from build123d import *

# Parameters (mm, degrees)
SKETCH1_W                      = 90
SKETCH1_H                      = 20
BOSS_EXTRUDE1_DEPTH            = 7
CBORE_START                    = 4
CBORE_FOR_M3_SHCS1_OUTLINE_R   = 3.25
CBORE_FOR_M3_SHCS1_DEPTH       = 3
CBORE_FOR_M3_SHCS1_2_OUTLINE_R = 1.7
CBORE_FOR_M3_SHCS1_2_DEPTH     = 4
SKETCH4_W                      = 70
SKETCH4_H                      = 16
CUT_EXTRUDE1_DEPTH             = 5
CHAMFER1_SIZE                  = 2
FILLET1_R                      = 2
CHAMFER2_SIZE                  = 2


# Read off the part's stored shape, not the designer's step: CBORE for M3 SHCS1
with BuildPart() as part:
    # Sketch1 → Boss-Extrude1 (new body)
    with BuildSketch(Plane(origin=(0, 0, 0), x_dir=(1, 0, 0), z_dir=(0, 1, 0))):
        Rectangle(SKETCH1_W, SKETCH1_H)
    extrude(amount=BOSS_EXTRUDE1_DEPTH)

    # CBORE for M3 SHCS1 outline → CBORE for M3 SHCS1 (cut)
    with BuildSketch(Plane(origin=(0, 0, 0), x_dir=(1, 0, 0), z_dir=(0, 1, 0)).offset(CBORE_START)):
        with Locations((-40, 0)):
            Circle(CBORE_FOR_M3_SHCS1_OUTLINE_R)
        with Locations((40, 0)):
            Circle(CBORE_FOR_M3_SHCS1_OUTLINE_R)
    extrude(amount=CBORE_FOR_M3_SHCS1_DEPTH, mode=Mode.SUBTRACT)

    # CBORE for M3 SHCS1 2 outline → CBORE for M3 SHCS1 2 (cut)
    with BuildSketch(Plane(origin=(0, 0, 0), x_dir=(1, 0, 0), z_dir=(0, 1, 0))):
        with Locations((-40, 0)):
            Circle(CBORE_FOR_M3_SHCS1_2_OUTLINE_R)
        with Locations((40, 0)):
            Circle(CBORE_FOR_M3_SHCS1_2_OUTLINE_R)
    extrude(amount=CBORE_FOR_M3_SHCS1_2_DEPTH, mode=Mode.SUBTRACT)

    # Sketch4 → Cut-Extrude1 (cut)
    with BuildSketch(Plane(origin=(0, 7, 0), x_dir=(1, 0, 0), z_dir=(0, 1, 0))):
        Rectangle(SKETCH4_W, SKETCH4_H)
    extrude(amount=-CUT_EXTRUDE1_DEPTH, mode=Mode.SUBTRACT)

    # Chamfer1
    chamfer1_edges = [part.edges().sort_by_distance(p)[0] for p in [
        (45, 3.5, 10),
        (-45, 3.5, 10),
        (-45, 3.5, -10),
        (45, 3.5, -10),
    ]]
    chamfer(chamfer1_edges, length=CHAMFER1_SIZE)

    # Fillet1
    fillet1_edges = [part.edges().sort_by_distance(p)[0] for p in [
        (-35, 4.5, -8),
        (-35, 4.5, 8),
        (35, 4.5, 8),
        (35, 4.5, -8),
    ]]
    fillet(fillet1_edges, radius=FILLET1_R)

    # Chamfer2
    chamfer2_edges = [part.edges().sort_by_distance(p)[0] for p in [
        (35, 2, 0),
        (0, 2, 8),
        (0, 2, -8),
        (-35, 2, 0),
        (-34.414213562, 2, 7.414213562),
        (-34.414213562, 2, -7.414213562),
        (34.414213562, 2, -7.414213562),
        (34.414213562, 2, 7.414213562),
    ]]
    chamfer(chamfer2_edges, length=CHAMFER2_SIZE)


solid = part.part
The listing builds one solid part. Answer for the finished solid, in the listing's coordinates (mm). A direction names the side the tool comes from. Give positions to 0.01 mm unless a question says otherwise; leave off trailing zeros. Order: outer loops, then holes, each group sorted by start corner. A loop starts at its lowest first (then second) coordinate and runs counter-clockwise, first axis right, second up. Notation, with made-up numbers: (-4, 5) -> (51, 5) arc R14 cw to (51, 31) -> close; hole circle Ø7 at (37.5, -26). An arc over 180 degrees is marked (long way). Put each result on its own line as item: value.
Item 1: For a pull along Z with two mould halves and no side action, classify faces 3 (the face through (0, 7, -9)), 4 (the face through (-1, 3, -10)), 5 (the face through (0, 3, -7)) as released by +Z, released by -Z, zero draft, split by the parting line, or undercut.
Established:
face 3: zero draft
face 4: released by -Z
face 5: undercut
Item 2: Straight lines are drawn through the part: line 1 (X direction, y = 5.25, z = 0); line 2 (X direction, y = 1.5, z = 0); line 3 (X direction, y = 3.75, z = 0.5). For each, find the intervals that lie inside material, in ascending order.
Established:
line 1: x = -45 to -43.25, -36.75 to -35, 35 to 36.75, 43.25 to 45
line 2: x = -45 to -41.7, -38.3 to 38.3, 41.7 to 45
line 3: x = -45 to -41.62, -38.38 to -34.75, 34.75 to 38.38, 41.62 to 45
Item 3: A cutting plane is placed at B-B on x = 40. Give the vertices of the cut face in (y, z), plus the area to 3 significant figures.
Established:
outline: (0, -10) -> (7, -10) -> (7, -3.25) -> (4, -3.25) -> (4, -1.7) -> (0, -1.7) -> close; (0, 1.7) -> (4, 1.7) -> (4, 3.25) -> (7, 3.25) -> (7, 10) -> (0, 10) -> close
area: 107 mm^2
Item 4: A cutting plane is placed at A-A on y = 2.75. Give the vertices of the cut face in (x, z), plus the area to 3 significant figures.
Established:
outline: (-45, -8) -> (-43, -10) -> (43, -10) -> (45, -8) -> (45, 8) -> (43, 10) -> (-43, 10) -> (-45, 8) -> close; hole circle Ø3.4 at (-40, 0); hole (-33.75, -6) arc R0.75 ccw to (-33, -6.75) -> (33, -6.75) arc R0.75 ccw to (33.75, -6) -> (33.75, 6) arc R0.75 ccw to (33, 6.75) -> (-33, 6.75) arc R0.75 ccw to (-33.75, 6) -> close; hole circle Ø3.4 at (40, 0)
area: 863 mm^2
Item 5: Given P1, Ø8, axis at x = 25.5, z = 3, coming from the +Y side; P2, Ø5, axis at x = 24, z = -2, coming from the -Y side; P3, Ø6, axis at x = 29, z = 0, coming from the +Y side; P4, Ø4, axis at x = -40, z = 0, coming from the +Y side, each flat-ended and moving along its own axis, determine where each tip first touches the part or whether it passes through.
Established:
P1: stops at y = 3
P2: stops at y = 0
P3: stops at y = 2
P4: stops at y = 4
Item 6: A cutting plane is placed at D-D on x = 26. Give the vertices of the cut face in (y, z).
Established:
outline: (0, -10) -> (7, -10) -> (7, -8) -> (4, -8) -> (2, -6) -> (2, 6) -> (4, 8) -> (7, 8) -> (7, 10) -> (0, 10) -> close
Item 7: For faces 1 (the face through (44, 3, 9)), 2 (the face through (-35, 6, 0)), determine the directions among +Z, -Z, +X, -X, +Y, -Y from which every point of the face is accessible in a straight line to the end or side of a thin tool.
Established:
face 1: +Z, +X, +Y, -Y
face 2: +Y
Item 8: A cutting plane is placed at C-C on z = 0. Give the vertices of the cut face in (x, y).
Established:
outline: (-45, 0) -> (-41.7, 0) -> (-41.7, 4) -> (-43.25, 4) -> (-43.25, 7) -> (-45, 7) -> close; (-38.3, 0) -> (38.3, 0) -> (38.3, 4) -> (36.75, 4) -> (36.75, 7) -> (35, 7) -> (35, 4) -> (33, 2) -> (-33, 2) -> (-35, 4) -> (-35, 7) -> (-36.75, 7) -> (-36.75, 4) -> (-38.3, 4) -> close; (41.7, 0) -> (45, 0) -> (45, 7) -> (43.25, 7) -> (43.25, 4) -> (41.7, 4) -> close
